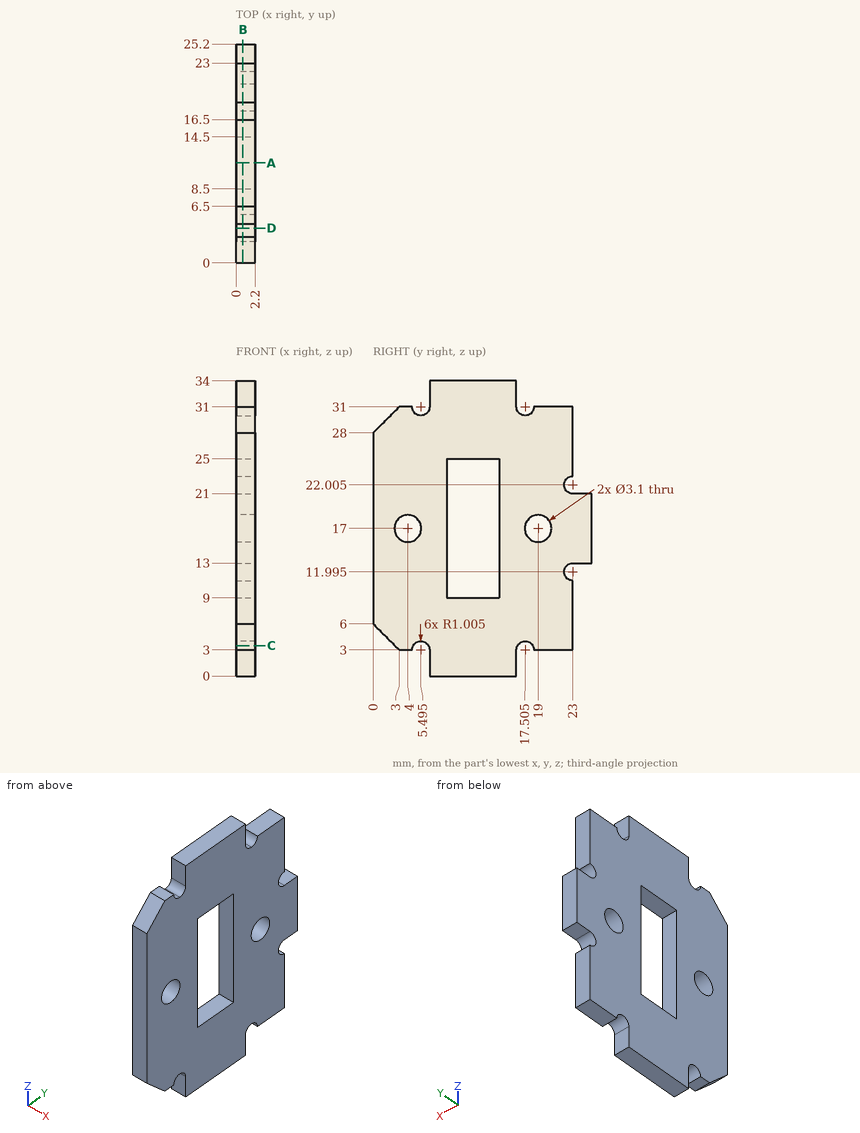
Here's the drawing with two shaded views (mm, measured from the low corner). I have some questions. Give positions to 0.01 mm unless a question says otherwise; leave off trailing zeros. Loops run counter-clockwise (first coordinate to the right, second up) from the corner with the lowest first, then second, coordinate; pieces in that order, holes last. Notation, with made-up numbers: M -8,71 L 27,71 A10 cw 27,90 Z; hole C 71,64 d11. An arc over 180 degrees is marked long. One line per item, written item: value.
1) Please list where these lines run through material, in increasing order: line 1 (Y direction, x = 1.35, z = 17); line 2 (Y direction, x = 1.3, z = 20); line 3 (Z direction, x = 0.9, y = 22.25).
Geometry check:
line 1: y = 0 to 2.45, 5.55 to 8.5, 14.5 to 17.45, 20.55 to 25.2
line 2: y = 0 to 8.5, 14.5 to 25.2
line 3: z = 3 to 11.33, 12.66 to 21.34, 22.67 to 31
2) Imagine slicing it at D-D on y = 4. Write out the boundary of the cut face in (x, z).
Geometry check:
outline: M 0,3 L 2.2,3 L 2.2,15.45 L 0,15.45 Z; M 0,18.55 L 2.2,18.55 L 2.2,31 L 0,31 Z
3) I'm going to push flat-ended pins straight in: pin 1 (1.1 mm diameter, centred on x = 1, z = 33, fed in from -Y); pin 2 (1.2 mm diameter, centred on x = 1.5, y = 3.5, fed in from +Z). Where does each tip first touch, or does it pass through?
Geometry check:
pin 1: stops at y = 6.5
pin 2: stops at z = 31
4) Imagine slicing it at C-C on z = 3.5. Write out the boundary of the cut face in (x, y).
Geometry check:
outline: M 0,2.5 L 2.2,2.5 L 2.2,4.62 L 0,4.62 Z; M 0,6.37 L 2.2,6.37 L 2.2,16.63 L 0,16.63 Z; M 0,18.38 L 2.2,18.38 L 2.2,23 L 0,23 Z
5) Imagine slicing it at A-A on y = 11.5. Write out the boundary of the cut face in (x, z), and give its area (3 significant figures).
Geometry check:
outline: M 0,0 L 2.2,0 L 2.2,9 L 0,9 Z; M 0,25 L 2.2,25 L 2.2,34 L 0,34 Z
area: 39.6 mm²
6) Imagine slicing it at B-B on x = 0.8. Count the separate pieces of the cut face and the enclosed holes in it, and give its area (3 significant figures).
Geometry check:
separate pieces: 1
enclosed holes: 3
area: 592 mm²
